```python
from build123d import *

# Parameters (mm, degrees)
SKETCH2_R               = 1.725
BOSS_EXTRUDE1_DEPTH     = 3.175
BOSS_EXTRUDE2_START     = 3.175
SKETCH2_3_R             = 1
BOSS_EXTRUDE2_DEPTH     = 6.35
CUT_EXTRUDE3_DEPTH      = 96.933443725
CUT_EXTRUDE3_DEPTH_BACK = 96.933443725


with BuildPart() as part:
    # Sketch2 → Boss-Extrude1 (new body)
    with BuildSketch(Plane.XY):
        Polygon((20, 20), (20, 67.5), (-20, 67.5), (-20, 20), (-67.5, 20), (-67.5, -20), (-20, -20), (-20, -67.5), (20, -67.5), (20, -20), (67.5, -20), (67.5, 20), align=None)
        with Locations((-10.253048327, 10.253048327)):
            Circle(SKETCH2_R, mode=Mode.SUBTRACT)
        Circle(SKETCH2_R, mode=Mode.SUBTRACT)
        with Locations((48.94, 0)):
            Circle(SKETCH2_R, mode=Mode.SUBTRACT)
        with Locations((-10.253048327, -10.253048327)):
            Circle(SKETCH2_R, mode=Mode.SUBTRACT)
    extrude(amount=BOSS_EXTRUDE1_DEPTH)

    # Sketch2<3> → Boss-Extrude2 (add)
    with BuildSketch(Plane.XY.offset(BOSS_EXTRUDE2_START)):
        with Locations((15, -57.6)):
            Circle(SKETCH2_3_R)
        with Locations((5, -57.6)):
            Circle(SKETCH2_3_R)
        with Locations((-5, -57.6)):
            Circle(SKETCH2_3_R)
        with Locations((-15, -57.6)):
            Circle(SKETCH2_3_R)
        with Locations((-15, -47.7)):
            Circle(SKETCH2_3_R)
        with Locations((-15, -37.8)):
            Circle(SKETCH2_3_R)
        with Locations((15, -37.8)):
            Circle(SKETCH2_3_R)
        with Locations((15, -47.7)):
            Circle(SKETCH2_3_R)
        with Locations((-15, -27.9)):
            Circle(SKETCH2_3_R)
        with Locations((15, -27.9)):
            Circle(SKETCH2_3_R)
        with Locations((-15, -18)):
            Circle(SKETCH2_3_R)
        with Locations((-18, -15)):
            Circle(SKETCH2_3_R)
        with Locations((-27.9, -15)):
            Circle(SKETCH2_3_R)
        with Locations((-37.8, -15)):
            Circle(SKETCH2_3_R)
        with Locations((-47.7, -15)):
            Circle(SKETCH2_3_R)
        with Locations((-57.6, -15)):
            Circle(SKETCH2_3_R)
        with Locations((-57.6, -5)):
            Circle(SKETCH2_3_R)
        with Locations((-57.6, 5)):
            Circle(SKETCH2_3_R)
        with Locations((-57.6, 15)):
            Circle(SKETCH2_3_R)
        with Locations((-47.7, 15)):
            Circle(SKETCH2_3_R)
        with Locations((-27.9, 15)):
            Circle(SKETCH2_3_R)
        with Locations((-18, 15)):
            Circle(SKETCH2_3_R)
        with Locations((-15, 18)):
            Circle(SKETCH2_3_R)
        with Locations((-15, 27.9)):
            Circle(SKETCH2_3_R)
        with Locations((-15, 37.8)):
            Circle(SKETCH2_3_R)
        with Locations((-15, 47.7)):
            Circle(SKETCH2_3_R)
        with Locations((-15, 57.6)):
            Circle(SKETCH2_3_R)
        with Locations((-5, 57.6)):
            Circle(SKETCH2_3_R)
        with Locations((5, 57.6)):
            Circle(SKETCH2_3_R)
        with Locations((15, 57.6)):
            Circle(SKETCH2_3_R)
        with Locations((15, 47.7)):
            Circle(SKETCH2_3_R)
        with Locations((15, 27.9)):
            Circle(SKETCH2_3_R)
        with Locations((15, 37.8)):
            Circle(SKETCH2_3_R)
        with Locations((15, 18)):
            Circle(SKETCH2_3_R)
        with Locations((18, 15)):
            Circle(SKETCH2_3_R)
        with Locations((27.9, 15)):
            Circle(SKETCH2_3_R)
        with Locations((37.8, 15)):
            Circle(SKETCH2_3_R)
        with Locations((47.7, 15)):
            Circle(SKETCH2_3_R)
        with Locations((57.6, 15)):
            Circle(SKETCH2_3_R)
        with Locations((57.6, 5)):
            Circle(SKETCH2_3_R)
        with Locations((57.6, -5)):
            Circle(SKETCH2_3_R)
        with Locations((57.6, -15)):
            Circle(SKETCH2_3_R)
        with Locations((47.7, -15)):
            Circle(SKETCH2_3_R)
        with Locations((37.8, -15)):
            Circle(SKETCH2_3_R)
        with Locations((15, -18)):
            Circle(SKETCH2_3_R)
        with Locations((18, -15)):
            Circle(SKETCH2_3_R)
        with Locations((27.9, -15)):
            Circle(SKETCH2_3_R)
        with Locations((-37.8, 15)):
            Circle(SKETCH2_3_R)
    extrude(amount=BOSS_EXTRUDE2_DEPTH)

    # Sketch3 → Cut-Extrude3 (cut, two sides: drawn at the far end of the back side and taken through both)
    with BuildSketch(Plane.XY.offset(-CUT_EXTRUDE3_DEPTH_BACK)):
        with BuildLine():
            Line((47.215, 0), (47.215, -52.394008893))
            ThreePointArc((47.215, -52.394008893), (48.94, -54.119008893), (50.665, -52.394008893))
            Line((50.665, -52.394008893), (50.665, 0))
            ThreePointArc((50.665, 0), (48.94, 1.725), (47.215, 0))
        make_face()
        with BuildLine():
            Line((-1.725, 0), (-1.725, -86.710184275))
            ThreePointArc((-1.725, -86.710184275), (0, -88.435184275), (1.725, -86.710184275))
            Line((1.725, -86.710184275), (1.725, 0))
            ThreePointArc((1.725, 0), (0, 1.725), (-1.725, 0))
        make_face()
        with BuildLine():
            Line((-11.978048327, 10.253048327), (-11.978048327, -86.719835381))
            ThreePointArc((-11.978048327, -86.719835381), (-10.253048327, -88.444835381), (-8.528048327, -86.719835381))
            Line((-8.528048327, -86.719835381), (-8.528048327, 10.253048327))
            ThreePointArc((-8.528048327, 10.253048327), (-10.253048327, 11.978048327), (-11.978048327, 10.253048327))
        make_face()
    extrude(amount=CUT_EXTRUDE3_DEPTH + CUT_EXTRUDE3_DEPTH_BACK, mode=Mode.SUBTRACT)


solid = part.part
```
For this review, take the finished solid that the model builds, in its own axes (mm). A direction names the side the tool comes from. Coordinates: 2 decimals unless noted, no trailing zeros. Order: outer loops, then holes, each group sorted by start corner. A loop starts at its lowest first (then second) coordinate and runs counter-clockwise, first axis right, second up. Notation, with made-up numbers: (-38.75, 18) - (-6.75, 18) arc R33 ccw to (-6.75, 47) - close; hole circle Ø8 at (79.25, 73). An arc over 180 degrees is marked (long way). Answer as a JSON object with one key per item and string values. Group by question number.
1. We need section B-B on z = 4.75. Give the number of separate pieces and of enclosed holes in the cut face, then the cut area to 3 significant figures.
2. For probe 1 along X at (y, z) = (-19.5, 3) (3 decimals); probe 2 along Y at (x, z) = (28, 3.25); probe 3 along X at (y, z) = (-25.5, 2.5) (3 decimals), list the stretches that pass through material, from the lowest coordinate up.
3. Clearance check with flat-ended pins moving along their axes: P1, Ø1.6, axis at y = -39, z = 1.5, coming from the -X side; P2, Ø4, axis at x = -24.5, z = 8, coming from the -Y side; P3, Ø1, axis at y = 52.5, z = 1.5, coming from the +X side; P4, Ø4, axis at x = -9.5, y = -23, coming from the -Z side. State where each tip first meets the part, or that it passes through.
4. We need section C-C on x = 24.5. State the section outline as (y, z) points (3 decimals), then the cut area to 3 significant figures.
5. The part is to be moulded in two halves that separate along Y. For faces 1 (the flat face through (-1, 16, 3.175)), 2 (the flat face through (-67.5, 0, 2)), 3 (the flat face through (44, 20, 2)), 4 (the cylindrical face through (0.038, 1.725, 1.565)), say which applies: pulls with the +Y half, pulls with the -Y half, needs draft (parallel to the pull), parting line crosses it, or undercut.
6. For faces 5 (the flat face through (11, -67.5, 2)), 6 (the flat face through (33, -20, 2)), 7 (the flat face through (-20, 44, 2)), 8 (the flat face through (-11.978, -28, 2)), 9 (the flat face through (-44, -20, 2)), list the 3-axis set-ups (+Z, -Z, +X, -X, +Y, -Y) from which the entire face can be reached by the end or side of a thin tool; tool diameter is ignored.
7. We need section A-A on y = -42. State the section outline as (x, z) points (3 decimals), then the cut area to 3 significant figures.
Final values:
{
 "1": {"separate pieces": "48", "enclosed holes": "0", "area": "148 mm²"},
 "2": {"probe 1": "-67.5 to -11.978, -8.528 to -1.725, 1.725 to 47.215, 50.665 to 67.5", "probe 2": "-15.99 to -14.01, 14.01 to 15.99", "probe 3": "-20 to -11.978, -8.528 to -1.725, 1.725 to 20"},
 "3": {"P1": "x = -20", "P2": "through", "P3": "x = 20", "P4": "z = 0"},
 "4": {"outline": "(-20, 0) - (20, 0) - (20, 3.175) - (-20, 3.175) - close", "area": "127 mm²"},
 "5": {"face 1": "undercut", "face 2": "needs draft", "face 3": "pulls with the +Y half", "face 4": "pulls with the -Y half"},
 "6": {"face 5": "+Z, -Z, +X, -X, -Y", "face 6": "+Z, -Z, +X, -Y", "face 7": "+Z, -Z, -X, +Y", "face 8": "+Z, -Z, -Y", "face 9": "+Z, -Z, -X, -Y"},
 "7": {"outline": "(-20, 0) - (-11.978, 0) - (-11.978, 3.175) - (-20, 3.175) - close; (-8.528, 0) - (-1.725, 0) - (-1.725, 3.175) - (-8.528, 3.175) - close; (1.725, 0) - (20, 0) - (20, 3.175) - (1.725, 3.175) - close", "area": "105 mm²"}
}
